For this review, take the finished solid that the model builds, in its own axes (mm). Face numbers are marked on the shaded views. Give positions to 0.01 mm unless a question says otherwise; leave off trailing zeros. Loops run counter-clockwise (first coordinate to the right, second up) from the corner with the lowest first, then second, coordinate; pieces in that order, holes last. Notation, with made-up numbers: (17.25, 41) - (69.25, 41) arc R34 cw to (69.25, 79) - close; hole circle Ø7 at (8.5, 79). An arc over 180 degrees is marked (long way). Put each result on its own line as item: value.
from build123d import *

# Parameters (mm, degrees)
SKETCH_1_W      = 200
SKETCH_1_H      = 200
EXTRUDE_1_DEPTH = 5
SKETCH_2_W      = 2.5
SKETCH_2_H      = 200
EXTRUDE_2_DEPTH = 20


with BuildPart() as part:
    # 草图1 → 凸台-拉伸1 (new body)
    with BuildSketch(Plane(origin=(0, 0, 0), x_dir=(1, 0, 0), z_dir=(0, 1, 0))):
        Rectangle(SKETCH_1_W, SKETCH_1_H)
    extrude(amount=EXTRUDE_1_DEPTH)

    # 草图2 → 凸台-拉伸2 (add)
    with BuildSketch(Plane.XZ):
        with Locations((-67.75, 0)):
            Rectangle(SKETCH_2_W, SKETCH_2_H)
        with Locations((-91.25, 0)):
            Rectangle(SKETCH_2_W, SKETCH_2_H)
    extrude_2 = extrude(amount=EXTRUDE_2_DEPTH)

    # 镜向1: 凸台-拉伸2 across plane
    add(extrude_2.mirror(Plane(origin=(0, 0, 0), x_dir=(0, 0, 1), z_dir=(1, 0, 0))))


solid = part.part
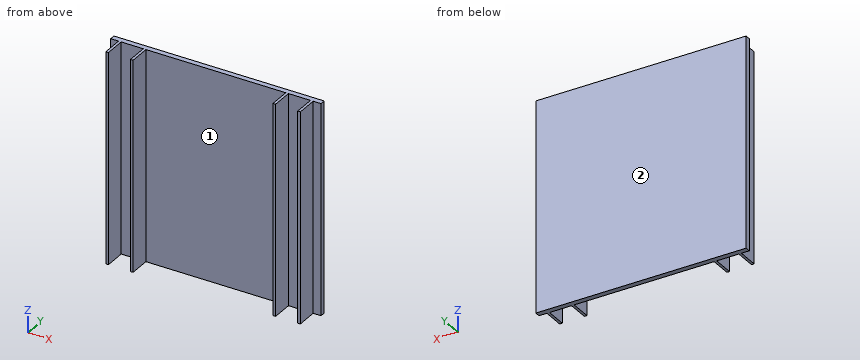
1) Take a section at A-A on y = -15.25. State the section outline as (x, z) points.
Geometry check:
outline: (-92.5, -100) - (-90, -100) - (-90, 100) - (-92.5, 100) - close; (-69, -100) - (-66.5, -100) - (-66.5, 100) - (-69, 100) - close; (66.5, -100) - (69, -100) - (69, 100) - (66.5, 100) - close; (90, -100) - (92.5, -100) - (92.5, 100) - (90, 100) - close
2) Wall thickness on line 1 (X direction, y = -13, z = 29.5); line 2 (Y direction, x = 80, z = -75): over which ranges is each line inside the solid? List them lowest first.
Geometry check:
line 1: x = -92.5 to -90, -69 to -66.5, 66.5 to 69, 90 to 92.5
line 2: y = 0 to 5
3) Insertion check: pin 1 Ø4 at (y, z) = (-14.5, 78.5) entering from -X; pin 2 Ø3 at (x, y) = (28.5, -1) entering from -Z; pin 3 Ø8 at (x, z) = (98, -0.5) entering from -Y; pin 4 Ø6 at (y, z) = (-12.5, -38.5) entering from +X. Each pin has a flat end and moves straight along its axis. Give the tip position at first contact, or say it passes through.
Geometry check:
pin 1: stops at x = -92.5
pin 2: stops at z = -100
pin 3: stops at y = 0
pin 4: stops at x = 92.5
4) Take a section at B-B on z = -39. State the section outline as (x, y) points, and give its area (3 significant figures).
Geometry check:
outline: (-100, 0) - (-92.5, 0) - (-92.5, -20) - (-90, -20) - (-90, 0) - (-69, 0) - (-69, -20) - (-66.5, -20) - (-66.5, 0) - (66.5, 0) - (66.5, -20) - (69, -20) - (69, 0) - (90, 0) - (90, -20) - (92.5, -20) - (92.5, 0) - (100, 0) - (100, 5) - (-100, 5) - close
area: 1,200 mm²
5) Take a section at C-C on x = 9. State the section outline as (y, z) points, and give its area (3 significant figures).
Geometry check:
outline: (0, -100) - (5, -100) - (5, 100) - (0, 100) - close
area: 1,000 mm²
6) Draft analysis for pull direction Y (two halves, no side actions). For the marked faces 1 and 2, state which applies: pulls with the +Y half, pulls with the -Y half, needs draft (parallel to the pull), parting line crosses it, or undercut.
Geometry check:
face 1: pulls with the -Y half
face 2: pulls with the +Y half
